from build123d import *

# Parameters (mm, degrees)
F1_DEPTH  = 1.5875
F3_DEPTH  = 4.7625
F4_W      = 6.35
F4_H      = 6.35
F5_DEPTH  = 3.175
F6_SIZE   = 1.8598642
F7_W      = 42.2204719395
F7_H      = 3.175
F8_DEPTH  = 1.5875
F9_W      = 6.35
F9_H      = 1.5875
F10_DEPTH = 6.35
F11_R     = 1.0922
F11_R_2   = 1.63322
F12_DEPTH = 28.575
F13_SIZE  = 1.58749
F14_R     = 0.396875
F15_DEPTH = 6.35
F16_R     = 1.63322
F17_DEPTH = 1.5875
F18_W     = 138.5852359697
F18_H     = 53.8887336135
F19_DEPTH = 7.9375
F20_W     = 1.5875
F20_H     = 3.175
F21_DEPTH = 1.5875
F22_R     = 0.396875
F23_DEPTH = 3.175


# Not quite as in the source:
# - a fillet or chamfer is up to 0.001 mm smaller than in the source, because OpenCascade refuses the exact size


with BuildPart() as f1:
    # F0 (on Top) → F1 (new body)
    with BuildSketch(Plane.XY):
        Polygon((-87.87765, 25.4), (-127, 25.4), (-127, 20.6375), (-48.7553, 20.6375), (-23.3553, -4.7625), (23.3553, -4.7625), (48.7553, 20.6375), (127, 20.6375), (127, 25.4), (87.87765, 25.4), (46.7826079092, 49.1262336135), (-46.7826079092, 49.1262336135), align=None)
        Polygon((-21.3826079092, 0), (-46.7826079092, 25.4), (-78.35265, 25.4), (-45.5064998802, 44.3637336135), (45.5064998802, 44.3637336135), (78.35265, 25.4), (46.7826079092, 25.4), (21.3826079092, 0), align=None, mode=Mode.SUBTRACT)
    extrude(amount=F1_DEPTH)

    # F2 (on face) → F3 (join)
    with BuildSketch(Plane.XY.offset(1.5875)):
        Polygon((-127, 22.225), (-127, 20.6375), (-48.7553, 20.6375), (-23.3553, -4.7625), (23.3553, -4.7625), (48.7553, 20.6375), (127, 20.6375), (127, 22.225), (93.376911314, 22.225), (87.87765, 25.4), (46.7826079092, 49.1262336135), (-46.7826079092, 49.1262336135), (-87.87765, 25.4), (-93.376911314, 22.225), align=None)
        Polygon((90.201911314, 22.225), (48.0977359697, 22.225), (22.6977359697, -3.175), (21.1102359697, -3.175), (21.1102359697, -1.5875), (-21.1102359697, -1.5875), (-21.1102359697, -3.175), (-22.6977359697, -3.175), (-48.0977359697, 22.225), (-90.201911314, 22.225), (-46.3572385662, 47.5387336135), (-21.1102359697, 47.5387336135), (-21.1102359697, 45.9512336135), (21.1102359697, 45.9512336135), (21.1102359697, 47.5387336135), (46.3572385662, 47.5387336135), align=None, mode=Mode.SUBTRACT)
    extrude(amount=F3_DEPTH)

    # F4 (on face) → F5 (join, through all)
    with BuildSketch(Plane(origin=(0, 22.225, 0), x_dir=(-1, 0, 0), z_dir=(0, 1, 0))):
        with Locations((-53.5178, 3.175)):
            Rectangle(F4_W, F4_H)
        with Locations((-123.825, 3.175)):
            Rectangle(F4_W, F4_H)
        with Locations((123.825, 3.175)):
            Rectangle(F4_W, F4_H)
        with Locations((53.5178, 3.175)):
            Rectangle(F4_W, F4_H)
    extrude(amount=F5_DEPTH)

    # F6
    f6_edges = [f1.edges().sort_by_distance(p)[0] for p in [
        (-127, 23.01875, 6.35),
        (-120.65, 23.8125, 6.35),
        (-56.6928, 23.8125, 6.35),
        (-50.3428, 23.8125, 6.35),
        (50.3428, 23.8125, 6.35),
        (56.6928, 23.8125, 6.35),
        (120.65, 23.8125, 6.35),
        (127, 23.01875, 6.35),
    ]]
    chamfer(f6_edges, length=F6_SIZE)

    # F7 (on face) → F8 (join)
    with BuildSketch(Plane.XY.offset(6.35)):
        with Locations((0, -3.175)):
            Rectangle(F7_W, F7_H)
        with Locations((0, 47.5387336135)):
            Rectangle(F7_W, F7_H)
    extrude(amount=F8_DEPTH)

    # F9 (on face) → F10 (cut, through all)
    with BuildSketch(Plane.XY.offset(7.9375)):
        with Locations((16.3477359697, -3.96875)):
            Rectangle(F9_W, F9_H)
        with Locations((16.3477359697, 48.3324836135)):
            Rectangle(F9_W, F9_H)
    extrude(amount=-F10_DEPTH, mode=Mode.SUBTRACT)

    # F11 (on face) → F12 (cut, through all)
    with BuildSketch(Plane.XZ.offset(3.175)):
        with Locations((53.5178, 3.175)):
            Circle(F11_R)
        with Locations((123.825, 3.175)):
            Circle(F11_R)
        with Locations((-123.825, 3.175)):
            Circle(F11_R)
        with Locations((-53.5178, 3.175)):
            Circle(F11_R)
        with Locations((16.3477359697, 4.7625)):
            Circle(F11_R_2)
    extrude(amount=-F12_DEPTH, mode=Mode.SUBTRACT)

    # F13 (size 1.5875 in the source; OpenCascade refuses exactly that, so slightly less here)
    f13_edges = [f1.edges().sort_by_distance(p)[0] for p in [
        (-21.110236, -3.96875, 6.35),
        (21.110236, -3.96875, 6.35),
        (-21.110236, 48.332484, 6.35),
        (21.110236, 48.332484, 6.35),
    ]]
    chamfer(f13_edges, length=F13_SIZE)

    # F14 (on face) → F15 (cut, through all)
    with BuildSketch(Plane.XY.offset(7.9375)):
        with Locations((19.5227359697, -3.175)):
            Circle(F14_R)
        with Locations((19.5227359697, 47.5387336135)):
            Circle(F14_R)
    extrude(amount=-F15_DEPTH, mode=Mode.SUBTRACT)

    # F16 (on face) → F17 (cut, through all)
    with BuildSketch(Plane(origin=(0, 47.5387336135, 0), x_dir=(-1, 0, 0), z_dir=(0, 1, 0))):
        with Locations((-16.3477359697, 4.7625)):
            Circle(F16_R)
    extrude(amount=-F17_DEPTH, mode=Mode.SUBTRACT)

    # F18 (on face) → F19 (cut, through all)
    with BuildSketch(Plane.XY.offset(7.9375)):
        with Locations((-57.7073820151, 22.1818668067)):
            Rectangle(F18_W, F18_H)
    extrude(amount=-F19_DEPTH, mode=Mode.SUBTRACT)

    # F20 (on face) → F21 (cut, through all)
    with BuildSketch(Plane.YZ.offset(13.1727359697)):
        with Locations((48.3324836135, 6.35)):
            Rectangle(F20_W, F20_H)
        with Locations((-3.96875, 6.35)):
            Rectangle(F20_W, F20_H)
    extrude(amount=-F21_DEPTH, mode=Mode.SUBTRACT)

    # F22 (on face) → F23 (cut, through all)
    with BuildSketch(Plane.XY.offset(4.7625)):
        with Locations((13.1727359697, -3.175)):
            Circle(F22_R)
        with Locations((13.1727359697, 47.5387336135)):
            Circle(F22_R)
    extrude(amount=-F23_DEPTH, mode=Mode.SUBTRACT)


solid = f1.part
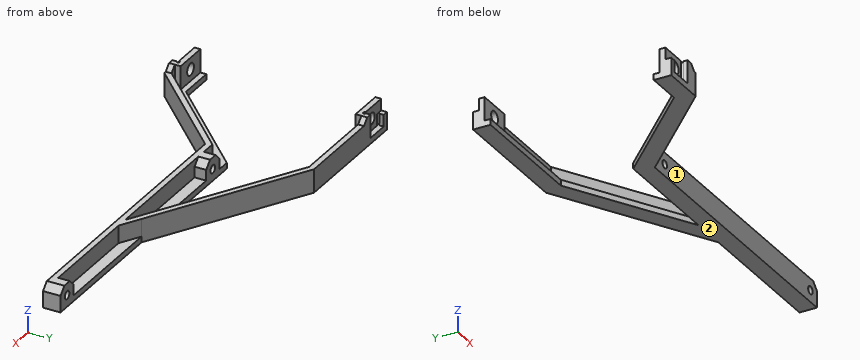
Source: CAD feature listing. Evaluate the final solid. Frame: model axes, mm. Face numbers are marked on the shaded views. A direction names the side the tool comes from. Give positions to 0.01 mm unless a question says otherwise; leave off trailing zeros. Write each loop counter-clockwise with the first axis right and the second up, starting at its lowest first coordinate (ties: lowest second). Pieces come first, ordered by that corner, then holes. Notation, with made-up numbers: (-23, 46) - (6, 46) arc R20 ccw to (6, 78) - close; hole circle Ø8 at (49.25, 79). An arc over 180 degrees is marked (long way). Write item = value, one per line. Start each with the question number.
Q1. Cut plane B-B, the plane y = 40.5. Return loops of the section in (x, z), then the cut area to 3 significant figures.
Q2. Reachability of the marked faces 1 and 2 from +Z, -Z, +X, -X, +Y, -Y: full face, straight path, thin tool, end or side. Return the list, or none.
Q3. Material intervals for probe 1 along Y at (x, z) = (121, 4); probe 2 along Z at (x, y) = (94.5, 23.5); probe 3 along X at (y, z) = (22.5, 5), sorted ascending.
Q4. Cut plane D-D, the plane x = 39. Return loops of the section in (y, z), then the cut area to 3 significant figures.
Q5. Pin query (flat end, axial travel): pin 1 Ø6 at (x, y) = (55, 40) entering from +Z; pin 2 Ø3 at (y, z) = (4.5, 3.5) entering from +X; pin 3 Ø1.7 at (x, z) = (31, 1) entering from -Y; pin 4 Ø2 at (x, z) = (123.825, 3.175) entering from -Y. Return the tip coordinate at first contact, or that it passes through.
Computed values:
q1.outline = (52.2, 0) - (61.72, 0) - (61.72, 6.35) - (58.55, 6.35) - (58.55, 1.59) - (52.2, 1.59) - close
q1.area = 30.2 mm²
q2.face_1 = +Z, -Z, +X, -Y
q2.face_2 = -Z, +X, -X, +Y, -Y
q3.probe_1 = 20.64 to 25.4
q3.probe_2 = 0 to 1.59
q3.probe_3 = 50.85 to 56.18, 89.73 to 92.9, 121.16 to 126.49
q4.outline = (10.88, 0) - (17.62, 0) - (17.62, 1.59) - (13.13, 1.59) - (13.13, 6.35) - (10.88, 6.35) - close; (44.36, 0) - (49.13, 0) - (49.13, 6.35) - (47.54, 6.35) - (47.54, 1.59) - (44.36, 1.59) - close
q4.area = 36.5 mm²
q5.pin_1 = 6.35
q5.pin_2 = 34.12
q5.pin_3 = 2.03
q5.pin_4 = through
